```python
from build123d import *

# Parameters (mm, degrees)
BOSS_EXTRUDE1_START                              = -2
BOSS_EXTRUDE1_OUTLINE_R                          = 27.3625
BOSS_EXTRUDE1_DEPTH                              = 2
BOSS_EXTRUDE1_2_DEPTH                            = 0.2
BOSS_EXTRUDE1_3_OUTLINE_R                        = 28.575
BOSS_EXTRUDE1_3_OUTLINE_R_2                      = 27.3625
BOSS_EXTRUDE1_3_DEPTH                            = 1
SKETCH2_W                                        = 2.2
SKETCH2_H                                        = 28.956
CUT_EXTRUDE1_DEPTH                               = 5.723285802
BOSS_EXTRUDE2_DEPTH                              = 1.8
CUT_EXTRUDE2_START                               = -2
CUT_EXTRUDE2_DEPTH                               = 2
CUT_EXTRUDE3_START                               = -2
CUT_EXTRUDE3_DEPTH                               = 2
SKETCH6_W                                        = 5
SKETCH6_H                                        = 2.2
F_11_0_11_DIAMETER_HOLE1_D                       = 11
F_11_0_11_DIAMETER_HOLE2_D                       = 11
F_11_0_11_DIAMETER_HOLE2_DEPTH                   = 4.8
F_2_4_2_4_DIAMETER_HOLE1_D                       = 2.4
CBORE_FOR_M4_HEX_HEAD_MACHINE_SCREW1_D           = 4.4
CBORE_FOR_M4_HEX_HEAD_MACHINE_SCREW1_CBORE_D     = 7.62
CBORE_FOR_M4_HEX_HEAD_MACHINE_SCREW1_CBORE_DEPTH = 2.032
FILLET1_R                                        = 1
SKETCH17_W                                       = 10.432207601
SKETCH17_H                                       = 12.73580757
BOSS_EXTRUDE3_DEPTH                              = 10
SKETCH18_R                                       = 1.5
BOSS_EXTRUDE4_DEPTH                              = 10


with BuildPart() as part:
    # Boss-Extrude1: read off the stored shape, not the designer's step
    # Boss-Extrude1 outline → Boss-Extrude1 (new body)
    with BuildSketch(Plane.XY.offset(2).offset(BOSS_EXTRUDE1_START)):
        Circle(BOSS_EXTRUDE1_OUTLINE_R)
        with BuildLine():
            Line((-1.524, -15.557918103), (-1.524, 12.7))
            Line((-1.524, 12.7), (2.912714198, 12.7))
            Line((2.912714198, 12.7), (2.912714198, -16.256))
            ThreePointArc((2.912714198, -16.256), (0.777149513, -15.38076538), (-1.524, -15.557918103))
        make_face(mode=Mode.SUBTRACT)
    extrude(amount=BOSS_EXTRUDE1_DEPTH)

    # Boss-Extrude1 2 outline → Boss-Extrude1 2 (add)
    with BuildSketch(Plane.XY.offset(2)):
        with BuildLine():
            ThreePointArc((2.912714198, -16.256), (0.541695497, -15.349430014), (-1.968941943, -15.723994384))
            ThreePointArc((-1.968941943, -15.723994384), (-2.456104545, -15.591784186), (-2.945777915, -15.714368556))
            ThreePointArc((-2.945777915, -15.714368556), (-9.352442215, -14.770348817), (-10.198398357, -8.35))
            Line((-10.198398357, -8.35), (-26.057319629, -8.35))
            ThreePointArc((-26.057319629, -8.35), (27.285112269, 2.056466564), (-27.014512882, 4.35))
            Line((-27.014512882, 4.35), (-10.198398357, 4.35))
            ThreePointArc((-10.198398357, 4.35), (-9.371903961, 10.750484649), (-2.994712748, 11.740802252))
            ThreePointArc((-2.994712748, 11.740802252), (-2.00956475, 11.765559549), (-1.524, 12.623088776))
            Line((-1.524, 12.623088776), (-1.524, 12.7))
            Line((-1.524, 12.7), (2.912714198, 12.7))
            Line((2.912714198, 12.7), (2.912714198, -16.256))
        make_face()
    extrude(amount=BOSS_EXTRUDE1_2_DEPTH)

    # Boss-Extrude1 3 outline → Boss-Extrude1 3 (add)
    with BuildSketch(Plane.XY.offset(2).offset(BOSS_EXTRUDE1_START)):
        Circle(BOSS_EXTRUDE1_3_OUTLINE_R)
        Circle(BOSS_EXTRUDE1_3_OUTLINE_R_2, mode=Mode.SUBTRACT)
    extrude(amount=BOSS_EXTRUDE1_3_DEPTH)

    # Sketch2 → Cut-Extrude1 (cut)
    with BuildSketch(Plane.ZY.offset(-2.912714198)):
        with Locations((1.1, -1.778)):
            Rectangle(SKETCH2_W, SKETCH2_H)
    extrude(amount=-CUT_EXTRUDE1_DEPTH, mode=Mode.SUBTRACT)

    # Sketch3 → Boss-Extrude2 (add)
    with BuildSketch(Plane.XY.offset(2.2)):
        with BuildLine():
            Line((-10.198398357, 4.35), (-27.014512882, 4.35))
            ThreePointArc((-27.014512882, 4.35), (27.285112269, 2.056466564), (-26.057319629, -8.35))
            Line((-26.057319629, -8.35), (-10.198398357, -8.35))
            ThreePointArc((-10.198398357, -8.35), (-9.352442215, -14.770348817), (-2.945777915, -15.714368556))
            ThreePointArc((-2.945777915, -15.714368556), (-2.109961399, -15.657248447), (-1.524001902, -16.256))
            Line((-1.524001902, -16.256), (8.636, -16.256))
            Line((8.636, -16.256), (8.636, 12.7))
            Line((8.636, 12.7), (-1.524, 12.7))
            Line((-1.524, 12.7), (-1.524, 12.623088776))
            ThreePointArc((-1.524, 12.623088776), (-2.00956475, 11.765559549), (-2.994712748, 11.740802252))
            ThreePointArc((-2.994712748, 11.740802252), (-9.371903961, 10.750484649), (-10.198398357, 4.35))
        make_face()
    extrude(amount=BOSS_EXTRUDE2_DEPTH)

    # Sketch4 → Cut-Extrude2 (cut)
    with BuildSketch(Plane.XY.offset(4).offset(CUT_EXTRUDE2_START)):
        with BuildLine():
            Line((-14.524, 4.35), (-10.198398357, 4.35))
            ThreePointArc((-10.198398357, 4.35), (-10.627065698, 5.317376904), (-10.857854141, 6.35))
            Line((-10.857854141, 6.35), (-12.524, 6.35))
            ThreePointArc((-12.524, 6.35), (-13.231106781, 6.057106781), (-13.524, 5.35))
            ThreePointArc((-13.524, 5.35), (-13.816893219, 4.642893219), (-14.524, 4.35))
        make_face()
    extrude(amount=CUT_EXTRUDE2_DEPTH, mode=Mode.SUBTRACT)

    # Sketch5 → Cut-Extrude3 (cut)
    with BuildSketch(Plane.XY.offset(4).offset(CUT_EXTRUDE3_START)):
        with BuildLine():
            Line((-12.524, -10.35), (-10.857854141, -10.35))
            ThreePointArc((-10.857854141, -10.35), (-10.627065698, -9.317376904), (-10.198398357, -8.35))
            Line((-10.198398357, -8.35), (-14.524, -8.35))
            ThreePointArc((-14.524, -8.35), (-13.816893219, -8.642893219), (-13.524, -9.35))
            ThreePointArc((-13.524, -9.35), (-13.231106781, -10.057106781), (-12.524, -10.35))
        make_face()
    extrude(amount=CUT_EXTRUDE3_DEPTH, mode=Mode.SUBTRACT)

    # Sketch6 → Cut-Revolve1 (revolve, cut)
    with BuildSketch(Plane.XZ.offset(20.32)):
        with Locations((2.5, 1.1)):
            Rectangle(SKETCH6_W, SKETCH6_H)
    revolve(axis=Axis((0, -20.32, 2.2), (0, 0, -1)), mode=Mode.SUBTRACT)

    # Sketch7 → Revolve1 (revolve)
    with BuildSketch(Plane(origin=(0, 22.86, 0), x_dir=(1, 0, 0), z_dir=(0, 1, 0))):
        with BuildLine():
            Line((4.154795897, -4), (0, -4))
            Line((0, -4), (0, -4.8))
            Line((0, -4.8), (3.175, -4.8))
            ThreePointArc((3.175, -4.8), (3.522340365, -4.225403331), (4.154795897, -4))
        make_face()
    revolve(axis=Axis((0, 22.86, 4), (0, 0, 1)))

    # Sketch8 → Revolve2 (revolve)
    with BuildSketch(Plane(origin=(0, 0, 0), x_dir=(1, 0, 0), z_dir=(0, 1, 0))):
        with BuildLine():
            Line((27.014795897, -4), (22.86, -4))
            Line((22.86, -4), (22.86, -4.8))
            Line((22.86, -4.8), (26.035, -4.8))
            ThreePointArc((26.035, -4.8), (26.382340365, -4.225403331), (27.014795897, -4))
        make_face()
    revolve(axis=Axis((22.86, 0, 4), (0, 0, 1)))

    # Ø11.0 (11) Diameter Hole1 (through all)
    with Locations(Plane.XY.offset(4)):
        with Locations((18.796, 8.89)):
            Hole(F_11_0_11_DIAMETER_HOLE1_D / 2)

    # Ø11.0 (11) Diameter Hole2
    with Locations(Plane(origin=(0, 0, 0), x_dir=(-1, 0, 0), z_dir=(0, 0, -1))):
        with Locations((18.796, 8.89)):
            Hole(F_11_0_11_DIAMETER_HOLE2_D / 2, depth=F_11_0_11_DIAMETER_HOLE2_DEPTH)

    # Ø2.4 (2.4) Diameter Hole1 (through all)
    with Locations(Plane.XY.offset(2)):
        with Locations((-5.524, 7), (-5.524, -11)):
            Hole(F_2_4_2_4_DIAMETER_HOLE1_D / 2)

    # CBORE for M4 Hex Head Machine Screw1 (through all)
    with Locations(Plane(origin=(0, 0, 0), x_dir=(-1, 0, 0), z_dir=(0, 0, -1))):
        with Locations((-22.86, 0), (0, 22.86)):
            CounterBoreHole(CBORE_FOR_M4_HEX_HEAD_MACHINE_SCREW1_D / 2, CBORE_FOR_M4_HEX_HEAD_MACHINE_SCREW1_CBORE_D / 2, CBORE_FOR_M4_HEX_HEAD_MACHINE_SCREW1_CBORE_DEPTH)

    # Fillet1
    fillet1_edges = [part.edges().sort_by_distance(p)[0] for p in [
        (3.556, 12.7, 4),
        (8.636, -1.778, 4),
        (3.555999049, -16.256, 4),
        (-10.857854141, -10.35, 3.1),
        (-10.857854141, 6.35, 3.1),
    ]]
    fillet(fillet1_edges, radius=FILLET1_R)

    # Sketch17 → Boss-Extrude3 (add)
    with BuildSketch(Plane.XY.offset(2)):
        with Locations((-6.740103801, -2)):
            Rectangle(SKETCH17_W, SKETCH17_H)
    extrude(amount=BOSS_EXTRUDE3_DEPTH)

    # Sketch18 → Boss-Extrude4 (add)
    with BuildSketch(Plane(origin=(-1.524, 0, 0), x_dir=(0, 0, -1), z_dir=(1, 0, 0))):
        with Locations(Location((-6.880774337, -2.000001215, 0), (0, 0, 90))):
            Circle(SKETCH18_R)
    extrude(amount=BOSS_EXTRUDE4_DEPTH)


solid = part.part
```
The listing builds one solid part. Answer for the finished solid, in the listing's coordinates (mm). A direction names the side the tool comes from. Coordinates: 2 decimals unless noted, no trailing zeros. Loops run counter-clockwise (first coordinate to the right, second up) from the corner with the lowest first, then second, coordinate; pieces in that order, holes last. Notation, with made-up numbers: M -15,84.25 L -3,84.25 A21 cw -3,88.25 Z; hole C 12,10.5 d3. An arc over 180 degrees is marked long. Answer as CSV lines item,"result". Start each with the question number.
(1) The part is cut by section A-A (x = 22.86). Give the vertices of the cut face in (y, z) (3 decimals), and give its area (3 significant figures).
(2) The part is cut by section D-D (y = -20.32). Give the vertices of the cut face in (x, z), and give its area (3 significant figures).
(3) Find the intervals of material crossed by L1, parallel to Y at x = 0, z = 1.1; L2, parallel to X at y = 4, z = 10.25; L3, parallel to Y at x = -4.5, z = 3.75, in increasing order. Write a range as [from, to].
(4) Given pin 1 (3 mm diameter, centred on x = 1, y = -22.5, fed in from -Z); pin 2 (1.5 mm diameter, centred on y = -2.5, z = 6.5, fed in from +X); pin 3 (3 mm diameter, centred on x = -9, z = 8.5, fed in from -Y); pin 4 (1.4 mm diameter, centred on x = -5.524, y = 7, fed in from -Z), each flat-ended and moving along its own axis, determine where each tip first touches the part or whether it passes through.
(5) For faces 3 (the flat face through (-20, -8.35, 3)), 4 (the cylindrical face through (-8.09, 11.72, 2.99)), 5 (the flat face through (0, -21, 2.2)), determine the directions among +Z, -Z, +X, -X, +Y, -Y from which every point of the face is accessible in a straight line to the end or side of a thin tool.
(6) The mould has two halves that part along Y. Classify faces 1 (the flat face through (8.476, -2, 7)), 2 (the cylindrical face through (0.83, 19.14, 1)): pulls with the +Y half, pulls with the -Y half, needs draft (parallel to the pull), parting line crosses it, or undercut.
(7) The part is cut by section B-B (y = 8.89). Give the vertices of the cut face in (x, z), and give its area (3 significant figures).
(8) The part is cut by section C-C (x = 15). Give the vertices of the cut face in (y, z), and give its area (3 significant figures).
Determined:
1,outline,"M -17.145,0 L -3.81,0 L -3.81,2.032 L -2.2,2.032 L -2.2,4.8 L -3.175,4.8 A1 cw -4.155,4 L -15.038,4 L -15.038,1 L -17.145,1 Z; M 2.2,2.032 L 3.81,2.032 L 3.81,0 L 5.184,0 L 5.184,4 L 4.155,4 A1 cw 3.175,4.8 L 2.2,4.8 Z; M 12.596,0 L 17.145,0 L 17.145,1 L 15.038,1 L 15.038,4 L 12.596,4 Z"
1,area,"72.7 mm2"
2,outline,"M -20.09,0 L -5,0 L -5,2.2 L 5,2.2 L 5,0 L 20.09,0 L 20.09,1 L 18.32,1 L 18.32,4 L -18.32,4 L -18.32,1 L -20.09,1 Z"
2,area,"128 mm2"
3,L1,"[-27.36, -25.32], [12.7, 19.05], [26.67, 27.36]"
3,L2,"[-11.96, -1.52]"
3,L3,"[-26.99, -16.27], [-8.37, 4.37], [12.27, 26.99]"
4,pin 1,"z = 2.2"
4,pin 2,"x = 8.48"
4,pin 3,"y = -8.37"
4,pin 4,"through"
5,face 3,"+Z, -X"
5,face 4,"+Z"
5,face 5,"-Z"
6,face 1,"needs draft"
6,face 2,"undercut"
7,outline,"M -27.16,0 L -24.3,0 L -24.3,4 L -25.88,4 L -25.88,1 L -27.16,1 Z; M -13.3,0 L -1.52,0 L -1.52,2 L -10.55,2 L -10.55,4 L -13.3,4 Z; M 8.64,0 L 13.3,0 L 13.3,4 L 9.64,4 A1 ccw 8.64,3 Z; M 24.3,0 L 27.16,0 L 27.16,1 L 25.88,1 L 25.88,4 L 24.3,4 Z"
7,area,"62.7 mm2"
8,outline,"M -24.32,0 L 4.91,0 L 4.91,4 L -22.88,4 L -22.88,1 L -24.32,1 Z; M 12.87,0 L 24.32,0 L 24.32,1 L 22.88,1 L 22.88,4 L 12.87,4 Z"
8,area,"154 mm2"
